Model file for the job. Use its own axes, mm. A direction names the side the tool comes from. Give positions to 0.01 mm unless a question says otherwise; leave off trailing zeros. Write each loop counter-clockwise with the first axis right and the second up, starting at its lowest first coordinate (ties: lowest second). Pieces come first, ordered by that corner, then holes. Notation, with made-up numbers: (67, 22.5) - (80, 22.5) arc R27 ccw to (80, 46.5) - close; hole circle Ø8 at (-21.5, -22). An arc over 180 degrees is marked (long way). Use a Markdown table: item, result. Add a question column.
Autodesk Inventor part; units mm, degrees
ref_plane "YZ Plane" through (0, 0, 0) normal (1, 0, 0) x (0, 1, 0)
ref_plane "XZ Plane" through (0, 0, 0) normal (0, 1, 0) x (-1, 0, 0)
ref_plane "XY Plane" through (0, 0, 0) normal (0, 0, 1) x (1, 0, 0)
sketch "Sketch1" plane through (0, 0, 0) normal (1, 0, 0) x (0, 1, 0)
  line L0 (70, 0) -> (-70, 0)
  line L1 (-70, 0) -> (-70, 100)
  line L2 (-70, 100) -> (-60, 100)
  line L3 (-60, 100) -> (-60, 110)
  line L4 (-60, 110) -> (-45, 110)
  line L5 (-45, 110) -> (-45, 95)
  line L6 (-45, 95) -> (-45, 95)
  line L7 (-45, 95) -> (-45, 35)
  line L8 (-45, 35) -> (45, 35)
  line L9 (45, 35) -> (45, 95)
  line L10 (45, 95) -> (45, 95)
  line L11 (45, 95) -> (45, 110)
  line L12 (45, 110) -> (60, 110)
  line L13 (60, 110) -> (60, 100)
  line L14 (60, 100) -> (70, 100)
  line L15 (70, 100) -> (70, 0)
  point P0 (0, 0)
  point P1 (0, 0)
  point P2 (0, 35)
  dimension "d15" = 90
  dimension "d16" = 110
  dimension "d17" = 10
  dimension "d20" = 35
  dimension "d21" = 15
  dimension "d22" = 15
  dimension "d23" = 15
  dimension "d24" = 10
  dimension "d25" = 10
  dimension "d26" = 135
  dimension "d27" = 135
  dimension "d28" = 90
extrude "Extrusion1" add sketch "Sketch1" against normal blind 1985
sketch "Sketch2" plane through (0, 0, 0) normal (1, 0, 0) x (0, 0, -1)
  line L0 (0, -70) -> (0, 70)
  line L1 (-110, 45) -> (-35, 45)
  line L2 (0, 25) -> (0, 45)
  line L3 (0, 70) -> (0, -70)
  line L4 (0, -70) -> (10, -70)
  line L5 (0, 55) -> (10, 55)
  line L6 (10, 55) -> (10, -70)
  line L7 (5, 55) -> (5, 30.8047) construction
  line L8 (0, 70) -> (-100, 70)
  line L9 (10, 55) -> (5, 70)
  line L10 (5, 70) -> (0, 55)
  point P0 (0, 0)
  point P1 (5, -70)
  point P2 (0, 55)
  dimension "d36" = 10
  dimension "d43" = 15
extrude "Extrusion2" add sketch "Sketch2" against normal up to surface (1985 mm away)
fillet "Fillet2" radius 5 1 edges at (-992.5, 70, -5)
equation "\"d22\" = d21"
equation "\"d25\" = d17"
properties part number "Zarge" material "Copper"
(1) Two-plate mould, pull along Y, no slides. Class faces 1 (the flat face through (-979, -1, 35)), 2 (the flat face through (-1985, -1, 24)), 3 (the flat face through (-979, 70, 51)): +Y half, -Y half, draft (parallel to the pull), parting line (faces both ways), or undercut.
(2) Band-saw the part on A-A (z = 66). Write the cut outline in (x, y), then the cut area to 4 significant figures.
(3) Flat gauge pins, fed straight in: pin 1 (3 mm diameter, centred on x = -1093.5, z = 106, fed in from +Y); pin 2 (1.5 mm diameter, centred on x = -451.5, y = -34, fed in from +Z); pin 3 (3 mm diameter, centred on x = -1348, z = 107.5, fed in from -Y). Where does each tip first touch, or does it go through?
(4) Probe probe 1 along Z at (x, y) = (-701.5, 55.5); probe 2 along Y at (x, z) = (-1518.5, 90.5); probe 3 along Z at (x, y) = (-692.5, -60.5). List the from-to ranges inside material, lowest first. Write a range as [from, to].
(5) Band-saw the part on B-B (x = -1597). Write the cut outline in (y, z).
(6) Band-saw the part on C-C (y = 12.5). Write the cut outline in (x, z).
(7) Which spindle directions (+Z, -Z, +X, -X, +Y, -Y) get a long thin tool onto all of the face, cutting with end or side? Do faces 4 (the flat face through (-979, -70, 44)), 5 (the flat face through (-979, -45, 73)). Say none if no direction does.
Model answer:
| question | item | result |
|---|---|---|
| 1 | face 1 | undercut |
| 1 | face 2 | draft |
| 1 | face 3 | +Y half |
| 2 | outline | (-1985, -70) - (0, -70) - (0, -45) - (-1985, -45) - close; (-1985, 45) - (0, 45) - (0, 70) - (-1985, 70) - close |
| 2 | area | 99,250 mm^2 |
| 3 | pin 1 | stops at y = 60 |
| 3 | pin 2 | stops at z = 35 |
| 3 | pin 3 | stops at y = -60 |
| 4 | probe 1 | z = [-9.83, -0.17], [0, 110] |
| 4 | probe 2 | y = [-70, -45], [45, 70] |
| 4 | probe 3 | z = [-10, 100] |
| 5 | outline | (-70, -10) - (55, -10) - (55.77, -9.74) arc R5 ccw to (55.77, -0.26) - (55, 0) - (70, 0) - (70, 100) - (60, 100) - (60, 110) - (45, 110) - (45, 35) - (-45, 35) - (-45, 110) - (-60, 110) - (-60, 100) - (-70, 100) - close |
| 6 | outline | (-1985, -10) - (0, -10) - (0, 35) - (-1985, 35) - close |
| 7 | face 4 | +Z, -Z, +X, -X, -Y |
| 7 | face 5 | +Z, +X, -X |
